Model file for the job. Use its own axes, mm. A direction names the side the tool comes from. Round coordinates to 2 decimals unless told otherwise and drop trailing zeros. Loops run counter-clockwise (first coordinate to the right, second up) from the corner with the lowest first, then second, coordinate; pieces in that order, holes last. Notation, with made-up numbers: M -10.75,-2.5 L 8.25,-2.5 A19 cw 8.25,23.5 Z; hole C 76,-32 d1. An arc over 180 degrees is marked long. Use a Markdown table: item, result. Add a question column.
Q1. Cut at B-B (y = 15). Give the cut face in (x, z), plus the area to 3 significant figures.
Q2. Tool access for faces 1 (the face through (3.1, 4.1, 3.3)), 2 (the face through (4, 0, 2)), 3 (the face through (5, 9, 2)): list every direction of +Z, -Z, +X, -X, +Y, -Y with a clear straight run to the whole face (end or side of a thin tool).
Q3. Cut at C-C (x = 7.75). Give the cut face in (y, z).
Q4. Probe line 1 (X direction, y = 5.5, z = 2.5); line 2 (X direction, y = 6.25, z = 1.85). List the from-to ranges inside material, lowest first. Write a range as from..to.
Q5. Cut at A-A (z = 1.05). Give the cut face in (x, y).
Q6. Pin check, flat tip, straight feed: pin 1 (1 mm diameter, centred on x = 3, y = 19, fed in from -Z). Stop position of the tip, or through.
Autodesk Inventor part; units mm, degrees
ref_plane "YZ Plane" through (0, 0, 0) normal (1, 0, 0) x (0, 1, 0)
ref_plane "XZ Plane" through (0, 0, 0) normal (0, 1, 0) x (-1, 0, 0)
ref_plane "XY Plane" through (0, 0, 0) normal (0, 0, 1) x (1, 0, 0)
sketch "Esquisse1" plane through (0, 0, 0) normal (0, 0, 1) x (1, 0, 0)
  line L0 (0, 0) -> (0, 23)
  line L1 (-2, 0) -> (12, 0)
  line L2 (0, -4.6) -> (0, 27.6)
  line L3 (0, 23) -> (5, 23)
  line L4 (5, 23) -> (9.1829, 21.0495)
  line L5 (9.1829, 21.0495) -> (10, 18)
  line L6 (10, 18) -> (5, 18)
  line L7 (5, 18) -> (5, 0)
  line L8 (0, 0) -> (5, 0)
  point P0 (0, 0)
  dimension "d8" = 5
  dimension "d9" = 5
  dimension "d10" = 75
  dimension "d12" = 130
  dimension "d13" = 18
  dimension "d14" = 5
  dimension "d24" = 5
extrude "Extrusion1" add sketch "Esquisse1" along normal blind 5
sketch "Esquisse3" plane through (0, 0, 0) normal (0, -1, 0) x (1, 0, 0)
  line L0 (0, 5) -> (5, 5)
  line L1 (0, 0) -> (0, 5)
  point P0 (2.5, 2.5)
  point P1 (2.5, 5)
  dimension "d15" = 2.5
  dimension "d16" = 2.5
hole "Perçage1" at (2.5, 0, 2.5) direction (0, 1, 0) diameter 2 depth 8 tip angle 118
properties part number "calle"
Checked values:
| question | item | result |
|---|---|---|
| 1 | outline | M 0,0 L 5,0 L 5,5 L 0,5 Z |
| 1 | area | 25.0 mm^2 |
| 2 | face 1 | -Y |
| 2 | face 2 | +Z, -Z, +X, -X, -Y |
| 2 | face 3 | +Z, -Z, +X, -Y |
| 3 | outline | M 18,0 L 21.72,0 L 21.72,5 L 18,5 Z |
| 4 | line 1 | x = 0..1.5, 3.5..5 |
| 4 | line 2 | x = 0..1.74, 3.26..5 |
| 5 | outline | M 0,0 L 5,0 L 5,18 L 10,18 L 9.18,21.05 L 5,23 L 0,23 Z |
| 6 | pin 1 | stops at z = 0 |
